Read the model definition and answer for the solid it produces. Units are mm, in the model's axes. Face numbers are marked on the shaded views. A direction names the side the tool comes from. Coordinates: 2 decimals unless noted, no trailing zeros. Write each loop counter-clockwise with the first axis right and the second up, starting at its lowest first coordinate (ties: lowest second). Pieces come first, ordered by that corner, then holes.
(1) Which of the six approach directions +Z, -Z, +X, -X, +Y, -Y give full straight-line access (tool end or side, diameter ignored) to the marked faces 1, 2, 3, 4 and 5?
(2) Straight lines are drawn through the part: line 1 along X through (y, z) = (8, 9.5); line 2 along X through (y, z) = (4.25, 6); line 3 along Z through (x, y) = (25, 12.25). For each, find the intervals that lie inside material, in ascending order.
(3) The part is cut by section A-A, the plane x = 27. Determine the outline of the cut face in (y, z), and give its area (3 significant figures).
(4) Given pin 1 (6 mm diameter, centred on x = 23, y = 10.5, fed in from -Z); pin 2 (4 mm diameter, centred on x = 33, y = 7, fed in from +Z), each flat-ended and moving along its own axis, determine where each tip first touches the part or whether it passes through.
(5) The part is cut by section B-B, the plane x = 11.5. Determine the outline of the cut face in (y, z), and give its area (3 significant figures).
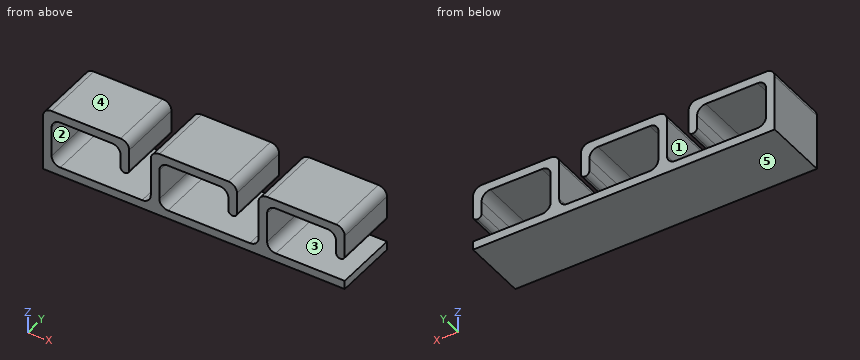
```python
from build123d import *

# Parameters (mm, degrees)
F1_DEPTH = 15
F2_R     = 2
F3_R     = 0.99999
F4_R     = 2


# Not quite as in the source:
# - a fillet or chamfer is up to 0.001 mm smaller than in the source, because OpenCascade refuses the exact size


with BuildPart() as f1:
    # F0 (on Front) → F1 (new body)
    with BuildSketch(Plane.XZ):
        Polygon((-12.5, 15), (-12.5, 0), (57.5, 0), (57.5, 2), (39.5, 2), (39.5, 13), (55.5, 13), (55.5, 7), (57.5, 7), (57.5, 15), (37.5, 15), (37.5, 2), (14.5, 2), (14.5, 13), (30.5, 13), (30.5, 7), (32.5, 7), (32.5, 15), (12.5, 15), (12.5, 2), (-10.5, 2), (-10.5, 13), (5.5, 13), (5.5, 7), (7.5, 7), (7.5, 15), align=None)
    extrude(amount=-F1_DEPTH)

    # F2
    f2_edges = [f1.edges().sort_by_distance(p)[0] for p in [
        (-10.5, 7.5, 2),
        (14.5, 7.5, 2),
        (39.5, 7.5, 2),
        (-10.5, 7.5, 13),
        (14.5, 7.5, 13),
        (39.5, 7.5, 13),
        (37.5, 7.5, 15),
        (12.5, 7.5, 15),
        (-12.5, 7.5, 15),
        (7.5, 7.5, 15),
        (32.5, 7.5, 15),
        (57.5, 7.5, 15),
        (5.5, 7.5, 13),
        (30.5, 7.5, 13),
        (55.5, 7.5, 13),
    ]]
    fillet(f2_edges, radius=F2_R)

    # F3 (radius 1 in the source; OpenCascade refuses exactly that, so slightly less here)
    f3_edges = [f1.edges().sort_by_distance(p)[0] for p in [
        (7.5, 7.5, 7),
        (5.5, 7.5, 7),
        (32.5, 7.5, 7),
        (30.5, 7.5, 7),
        (57.5, 7.5, 7),
        (55.5, 7.5, 7),
    ]]
    fillet(f3_edges, radius=F3_R)

    # F4
    f4_edges = [f1.edges().sort_by_distance(p)[0] for p in [
        (12.5, 7.5, 2),
        (37.5, 7.5, 2),
    ]]
    fillet(f4_edges, radius=F4_R)


solid = f1.part
```
Computed:
1. face 1: +Z, +Y, -Y
1. face 2: +Y, -Y
1. face 3: +X, +Y, -Y
1. face 4: +Z, +X, -X, +Y, -Y
1. face 5: -Z, +X, -X, +Y, -Y
2. line 1: x = -12.5 to -10.5, 5.5 to 7.5, 12.5 to 14.5, 30.5 to 32.5, 37.5 to 39.5, 55.5 to 57.5
2. line 2: x = -12.5 to -10.5, 12.5 to 14.5, 37.5 to 39.5
2. line 3: z = 0 to 2, 13 to 15
3. outline: (0, 0) - (15, 0) - (15, 2) - (0, 2) - close; (0, 13) - (15, 13) - (15, 15) - (0, 15) - close
3. area: 60.0 mm2
4. pin 1: stops at z = 0
4. pin 2: stops at z = 14.94
5. outline: (0, 0) - (15, 0) - (15, 2.27) - (0, 2.27) - close
5. area: 34.0 mm2
